from build123d import *

# Parameters (mm, degrees)
BOSS_EXTRUDE1_DEPTH = 63
SKETCH10_R          = 13
CUT_EXTRUDE3_DEPTH  = 70
SKETCH12_R          = 13
CUT_EXTRUDE4_DEPTH  = 70
SKETCH16_W          = 140
SKETCH16_H          = 27.398314348
CUT_EXTRUDE6_DEPTH  = 44
SKETCH17_R          = 13
CUT_EXTRUDE7_DEPTH  = 100
FILLET1_R           = 5
FILLET2_R           = 5
FILLET3_R           = 5
FILLET4_R           = 5
FILLET5_R           = 5
FILLET6_R           = 5
FILLET7_R           = 5
FILLET8_R           = 5


with BuildPart() as part:
    # Sketch2 → Boss-Extrude1 (new body)
    with BuildSketch(Plane.XY):
        Polygon((0, 0), (212, -3.51679799), (212, 21.48320201), (176, 21.48320201), (176, 65.48320201), (140, 65.48320201), (106, 38.193220771), (72, 69), (36, 69), (36, 25), (0, 25), align=None)
    extrude(amount=BOSS_EXTRUDE1_DEPTH)

    # Sketch10 → Cut-Extrude3 (cut)
    with BuildSketch(Plane(origin=(0, 0, 0), x_dir=(-1, 0, 0), z_dir=(0, 0, -1))):
        with Locations((-150.998263924, 46.995976699)):
            Circle(SKETCH10_R)
    extrude(amount=-CUT_EXTRUDE3_DEPTH, mode=Mode.SUBTRACT)

    # Sketch12 → Cut-Extrude4 (cut)
    with BuildSketch(Plane(origin=(0, 25, 0), x_dir=(1, 0, 0), z_dir=(0, 1, 0))):
        with Locations(Location((18, -31.5, 0), (0, 0, 270))):
            Circle(SKETCH12_R)
        with Locations((194, -31.5)):
            Circle(SKETCH12_R)
    extrude(amount=-CUT_EXTRUDE4_DEPTH, mode=Mode.SUBTRACT)

    # Sketch16 → Cut-Extrude6 (cut)
    with BuildSketch(Plane(origin=(0, 69, 0), x_dir=(1, 0, 0), z_dir=(0, 1, 0))):
        with Locations((106, -31.506588427)):
            Rectangle(SKETCH16_W, SKETCH16_H)
    extrude(amount=-CUT_EXTRUDE6_DEPTH, mode=Mode.SUBTRACT)

    # Sketch17 → Cut-Extrude7 (cut)
    with BuildSketch(Plane.XY.offset(63)):
        with Locations((60.97435617, 46.978804013)):
            Circle(SKETCH17_R)
    extrude(amount=-CUT_EXTRUDE7_DEPTH, mode=Mode.SUBTRACT)

    # Fillet1
    fillet1_edges = [part.edges().sort_by_distance(p)[0] for p in [
        (106, 38.193220771, 8.903715627),
    ]]
    fillet(fillet1_edges, radius=FILLET1_R)

    # Fillet2
    fillet2_edges = [part.edges().sort_by_distance(p)[0] for p in [
        (106, 38.193220771, 54.102872801),
    ]]
    fillet(fillet2_edges, radius=FILLET2_R)

    # Fillet3
    fillet3_edges = [part.edges().sort_by_distance(p)[0] for p in [
        (212, 21.48320201, 31.5),
    ]]
    fillet(fillet3_edges, radius=FILLET3_R - 0.0001)  # a hair under: the kernel refuses the full size

    # Fillet4
    fillet4_edges = [part.edges().sort_by_distance(p)[0] for p in [
        (176, 65.48320201, 54.102872801),
    ]]
    fillet(fillet4_edges, radius=FILLET4_R)

    # Fillet5
    fillet5_edges = [part.edges().sort_by_distance(p)[0] for p in [
        (176, 65.48320201, 8.903715627),
    ]]
    fillet(fillet5_edges, radius=FILLET5_R)

    # Fillet6
    fillet6_edges = [part.edges().sort_by_distance(p)[0] for p in [
        (36, 69, 54.102872801),
    ]]
    fillet(fillet6_edges, radius=FILLET6_R)

    # Fillet7
    fillet7_edges = [part.edges().sort_by_distance(p)[0] for p in [
        (36, 69, 8.903715627),
    ]]
    fillet(fillet7_edges, radius=FILLET7_R)

    # Fillet8
    fillet8_edges = [part.edges().sort_by_distance(p)[0] for p in [
        (0, 25, 31.5),
    ]]
    fillet(fillet8_edges, radius=FILLET8_R - 0.0001)  # a hair under: the kernel refuses the full size


solid = part.part
Check sheet for the modelled part. Datum: model origin and axes. Units: mm. A direction names the side the tool comes from. Give positions to 0.01 mm unless a question says otherwise; leave off trailing zeros. Write each loop counter-clockwise with the first axis right and the second up, starting at its lowest first coordinate (ties: lowest second). Pieces come first, ordered by that corner, then holes. Notation, with made-up numbers: (7, 63) -> (27, 63) arc R18 ccw to (27, 81) -> close; hole circle Ø7 at (46.25, -32.5). An arc over 180 degrees is marked (long way). Use one line per item in the form item = value. Start each with the question number.
1. Access from +Z, -Z, +X, -X, +Y, -Y to the whole of each face (thin tool, end or side, straight path). Record for faces 4 (the flat face through (124.878, 53.345, 8.779)), 5 (the flat face through (36, 45, 9)), 6 (the flat face through (156, 65.483, 9)).
2. Section check B-B (y = 6.5). Record the cut outline in (x, z).
3. Section check A-A (x = 51). Record the cut outline in (y, z).
4. Thickness scan on line 1 along X through (y, z) = (5, 31); line 2 along X through (y, z) = (17.5, 42); line 3 along Z through (x, y) = (82.5, 55). Record the ranges inside material, lowest first. Write a range as from..to.
5. Section check C-C (z = 31.5). Count the separate pieces of the cut face and the enclosed holes in it, and give its area (3 significant figures).
6. Section check D-D (x = 194). Record the cut outline in (y, z).
7. Go/stop test with flat-tipped pins: P1, Ø6, axis at y = 28.5, z = 48.5, coming from the +X side; P2, Ø15.5, axis at x = 187.5, z = 20, coming from the +Y side; P3, Ø3, axis at x = 38.5, z = 9, coming from the -Y side; P4, Ø10, axis at x = 40, z = 45.5, coming from the +Y side. Record where each tip stops, or that it passes through.
8. Mould release check, pull along X, two halves, no side actions. Record for faces 1 (the flat face through (124.878, 53.345, 53.978)), 2 (the cylindrical face through (174.574, 63.98, 54.227)), 3 (the flat face through (181, 21.483, 24)): pulls with the +X half, pulls with the -X half, needs draft (parallel to the pull), parting line crosses it, or undercut.
Conclusion:
q1.face_4 = +Z, -Z, +Y
q1.face_5 = +Z, -Z, -X, +Y
q1.face_6 = +Z, -Z, +X, +Y
q2.outline = (0, 0) -> (212, 0) -> (212, 63) -> (0, 63) -> close; hole circle Ø26 at (18, 31.5); hole circle Ø26 at (194, 31.5)
q3.outline = (-0.85, 0) -> (38.64, 0) -> (38.64, 17.81) -> (25, 17.81) -> (25, 45.21) -> (38.64, 45.21) -> (38.64, 63) -> (-0.85, 63) -> close; (55.32, 0) -> (69, 0) -> (69, 17.81) -> (55.32, 17.81) -> close; (55.32, 45.21) -> (69, 45.21) -> (69, 63) -> (55.32, 63) -> close
q4.line_1 = 0..5.01, 30.99..181.01, 206.99..212
q4.line_2 = 0..10.34, 25.66..186.34, 201.66..211.9
q4.line_3 = 0..17.81, 45.21..63
q5.separate_pieces = 3
q5.enclosed_holes = 0
q5.area = 4,240 mm²
q6.outline = (-3.22, 0) -> (21.48, 0) -> (21.48, 18.5) -> (-3.22, 18.5) -> close; (-3.22, 44.5) -> (21.48, 44.5) -> (21.48, 63) -> (-3.22, 63) -> close
q7.P1 = 176
q7.P2 = 21.48
q7.P3 = -0.66
q7.P4 = 69
q8.face_1 = undercut
q8.face_2 = pulls with the +X half
q8.face_3 = needs draft
